Here's how the part is built. I have some questions about the finished solid (model axes, mm). A direction names the side the tool comes from. Coordinates: 2 decimals unless noted, no trailing zeros. Write each loop counter-clockwise with the first axis right and the second up, starting at its lowest first coordinate (ties: lowest second). Pieces come first, ordered by that corner, then holes.
(1) Imagine slicing it at D-D, the plane y = 40. List the corners of the cut face in (x, z) for me.
(2) Imagine slicing it at C-C, the plane y = 24. List the corners of the cut face in (x, z) for me, plus the area to 3 significant figures.
(3) For pin 1 Ø4 at (x, z) = (12.22, -4.45) entering from +Y; pin 2 Ø1.5 at (x, y) = (-23.5, 37) entering from +Z, each with a flat end and sliding along its axis, tell me the tip position at first contact or that it passes through.
(4) Thinking about a two-plate mould opening in Z: for faces 1 (the cylindrical face through (-7.025, 42.521, -10.238)), 2 (the flat face through (14, 0, 9)), 3 (the cylindrical face through (10.238, 42.521, -7.025)), 4 (the cylindrical face through (-0.475, 21.692, 39.247)), which applies, released by +Z, released by -Z, zero draft, split by the parting line, or undercut?
(5) Imagine slicing it at B-B, the plane z = 0. List the corners of the cut face in (x, y) for me.
(6) Imagine slicing it at A-A, the plane x = 0. List the corners of the cut face in (y, z) for me.
(7) Please list where these lines run through material, in increasing order: probe 1 along X at (y, z) = (19.5, 0); probe 2 along Y at (x, z) = (1.5, 12); probe 3 along X at (y, z) = (4, 6.5).
(8) Which directions (+Z, -Z, +X, -X, +Y, -Y) give clear straight access to the entire face, cutting with the end or side of a thin tool? Please do faces 5 (the flat face through (-3, 41, -11)), 6 (the cylindrical face through (0.475, 21.692, -39.247)), 7 (the flat face through (-7, 35, -7)).
```python
from build123d import *

# Parameters (mm, degrees)
BOSS_EXTRUDE1_DEPTH            = 44
CBORE_FOR_M3_SHCS1_D           = 3.4
CBORE_FOR_M3_SHCS1_CBORE_D     = 6.5
CBORE_FOR_M3_SHCS1_CBORE_DEPTH = 3
CIRPATTERN1_COUNT              = 4
SKETCH4_R                      = 16.2
CUT_EXTRUDE1_DEPTH             = 35
SKETCH5_R                      = 9.7
CUT_EXTRUDE2_DEPTH             = 66.498740446
BOSS_EXTRUDE2_DEPTH            = 44


with BuildPart() as part:
    # Sketch1 → Boss-Extrude1 (new body)
    with BuildSketch(Plane(origin=(0, 0, 0), x_dir=(1, 0, 0), z_dir=(0, 1, 0))):
        with BuildLine():
            Line((-29.85, 23.917357714), (-29.85, -23.917357714))
            ThreePointArc((-29.85, -23.917357714), (0, -38.25), (29.85, -23.917357714))
            Line((29.85, -23.917357714), (29.85, 23.917357714))
            ThreePointArc((29.85, 23.917357714), (0, 38.25), (-29.85, 23.917357714))
        make_face()
    extrude(amount=BOSS_EXTRUDE1_DEPTH)

    # CBORE for M3 SHCS1 (through all)
    with Locations(Plane(origin=(0, 44, 0), x_dir=(1, 0, 0), z_dir=(0, 1, 0))):
        with Locations((-4.446261863, 12.21600407)):
            cbore_for_m3_shcs1 = CounterBoreHole(CBORE_FOR_M3_SHCS1_D / 2, CBORE_FOR_M3_SHCS1_CBORE_D / 2, CBORE_FOR_M3_SHCS1_CBORE_DEPTH)

    # CirPattern1: CBORE for M3 SHCS1 ×4 about axis
    cirpattern1_axis = Axis((0, 0, 0), (0, 1, 0))
    for i in range(1, CIRPATTERN1_COUNT):
        add(cbore_for_m3_shcs1.rotate(cirpattern1_axis, i * 360 / CIRPATTERN1_COUNT), mode=Mode.SUBTRACT)

    # Sketch4 → Cut-Extrude1 (cut)
    with BuildSketch(Plane.XZ):
        with Locations(Location((0, 0, 0), (0, 0, 270))):
            Circle(SKETCH4_R)
    extrude(amount=-CUT_EXTRUDE1_DEPTH, mode=Mode.SUBTRACT)

    # Sketch5 → Cut-Extrude2 (cut, through all)
    with BuildSketch(Plane(origin=(0, 44, 0), x_dir=(1, 0, 0), z_dir=(0, 1, 0))):
        with Locations(Location((0, 0, 0), (0, 0, 270))):
            Circle(SKETCH5_R)
    extrude(amount=-CUT_EXTRUDE2_DEPTH, mode=Mode.SUBTRACT)

    # Sketch7 → Boss-Extrude2 (add)
    with BuildSketch(Plane.XZ):
        with BuildLine():
            Line((-29.85, 23.917357714), (-29.85, 25.486074629))
            ThreePointArc((-29.85, 25.486074629), (0, 39.25), (29.85, 25.486074629))
            Line((29.85, 25.486074629), (29.85, 23.917357714))
            ThreePointArc((29.85, 23.917357714), (0, 38.25), (-29.85, 23.917357714))
        make_face()
        with BuildLine():
            Line((29.85, -23.917357714), (29.85, -25.486074629))
            ThreePointArc((29.85, -25.486074629), (0, -39.25), (-29.85, -25.486074629))
            Line((-29.85, -25.486074629), (-29.85, -23.917357714))
            ThreePointArc((-29.85, -23.917357714), (0, -38.25), (29.85, -23.917357714))
        make_face()
    extrude(amount=-BOSS_EXTRUDE2_DEPTH)


solid = part.part
```
Recorded:
1. outline: (-29.85, -25.49) arc R39.25 ccw to (29.85, -25.49) - (29.85, 25.49) arc R39.25 ccw to (-29.85, 25.49) - close; hole circle Ø3.4 at (-12.22, 4.45); hole circle Ø19.4 at (0, 0); hole circle Ø3.4 at (-4.45, -12.22); hole circle Ø3.4 at (4.45, 12.22); hole circle Ø3.4 at (12.22, -4.45)
2. outline: (-29.85, -25.49) arc R39.25 ccw to (29.85, -25.49) - (29.85, 25.49) arc R39.25 ccw to (-29.85, 25.49) - close; hole circle Ø32.4 at (0, 0)
2. area: 3,360 mm2
3. pin 1: stops at y = 41
3. pin 2: stops at z = 31.98
4. face 1: undercut
4. face 2: zero draft
4. face 3: undercut
4. face 4: released by +Z
5. outline: (-29.85, 0) - (-16.2, 0) - (-16.2, 35) - (-9.7, 35) - (-9.7, 44) - (-29.85, 44) - close; (9.7, 35) - (16.2, 35) - (16.2, 0) - (29.85, 0) - (29.85, 44) - (9.7, 44) - close
6. outline: (0, -39.25) - (44, -39.25) - (44, -9.7) - (35, -9.7) - (35, -16.2) - (0, -16.2) - close; (0, 16.2) - (35, 16.2) - (35, 9.7) - (44, 9.7) - (44, 39.25) - (0, 39.25) - close
7. probe 1: x = -29.85 to -16.2, 16.2 to 29.85
7. probe 2: y = 35 to 41
7. probe 3: x = -29.85 to -14.84, 14.84 to 29.85
8. face 5: +Y
8. face 6: -Z, +Y, -Y
8. face 7: -Y
